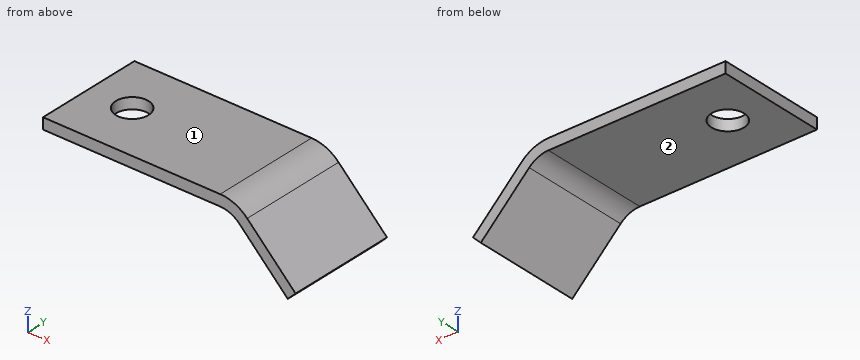
Autodesk Inventor part; units mm, degrees
ref_plane "YZ Plane" through (0, 0, 0) normal (1, 0, 0) x (0, 1, 0)
ref_plane "XZ Plane" through (0, 0, 0) normal (0, 1, 0) x (-1, 0, 0)
ref_plane "XY Plane" through (0, 0, 0) normal (0, 0, 1) x (1, 0, 0)
sketch "Sketch1" plane through (0, 0, 0) normal (0, 1, 0) x (-1, 0, 0)
  line L0 (0, 0) -> (-5.4801, -5.4801)
  line L1 (0, 0) -> (17.75, 0)
  dimension "d0" = 7.75
  dimension "d2" = 17.75
  dimension "d3" = 135
contour flange "Contour Flange1" sketch "Sketch1" thickness 1.016 bend radius 2.5 width 10 along (0, 1, 0) mid plane no both sides no wall seen from (2.74, 0, -2.74) lies toward (-0.7071068, 0, -0.7071068) curves L0 L1
bend "Bend1"
corner "Corner1"
sketch "Sketch2" plane through (-17.75, 0, -1.016) normal (0, 0, -1) x (-1, 0, 0)
  point P0 (-17.75, 0)
  point P1 (0, 0)
  point P2 (-4, 5)
  dimension "d15" = 5
  dimension "d16" = 4
hole "Hole1" at (-13.75, 5, -1.016) direction (0, 0, 1) diameter 3 end through all
equation "\"d22\" = Thickness"
equation "\"d4\" = Thickness"
equation "\"d5\" = BendReliefWidth"
equation "\"d6\" = BendReliefDepth"
equation "\"d7\" = MinimumRemnant"
equation "\"d8\" = TransitionRadius"
equation "\"d12\" = CornerReliefSize"
equation "\"d13\" = GapSize"
equation "\"d14\" = JacobiRadiusSize"
equation "\"BendRadius\" = Thickness"
equation "\"BendReliefWidth\" = Thickness"
equation "\"BendReliefDepth\" = 0.5 * Thickness"
equation "\"CornerReliefSize\" = 4 * Thickness"
equation "\"MinimumRemnant\" = 2 * Thickness"
equation "\"TransitionRadius\" = BendRadius"
equation "\"JacobiRadiusSize\" = BendRadius"
equation "\"GapSize\" = Thickness"
properties part number "Piston Flag" material "ABS Plastic"
Can you work these out from the model? Positions are in its coordinate system, mm. Face numbers are marked on the shaded views. A direction names the side the tool comes from. Coordinates: 2 decimals unless noted, no trailing zeros. Loops run counter-clockwise (first coordinate to the right, second up) from the corner with the lowest first, then second, coordinate; pieces in that order, holes last. Notation, with made-up numbers: (8.5, 72) - (51.5, 72) arc R14 ccw to (51.5, 82) - close; hole circle Ø6 at (-18.75, 24.25). An arc over 180 degrees is marked (long way). Answer as CSV lines item,"result". Start each with the question number.
1) Which directions (+Z, -Z, +X, -X, +Y, -Y) give clear straight access to the entire face, cutting with the end or side of a thin tool? Please do the marked faces 1 and 2.
2) Suppose I cut it at D-D (z = -3.25). Please give me the cut outline in (x, y).
3) Suppose I cut it at A-A (y = 5). Please give me the cut outline in (x, z), plus the area to 3 significant figures.
4) Suppose I cut it at B-B (x = -13.75). Please give me the cut outline in (y, z), plus the area to 3 significant figures.
5) For pin 1 (1.8 mm diameter, centred on x = -13.75, y = 5, fed in from +Z); pin 2 (1 mm diameter, centred on x = -11.5, y = 7.5, fed in from +Z); pin 3 (6 mm diameter, centred on x = -5, y = 2.5, fed in from -Z); pin 4 (2 mm diameter, centred on x = 1, y = 6, fed in from +Z), each with a flat end and sliding along its axis, tell me the tip position at first contact or that it passes through.
6) I need wall thicknesses on line 1 (Y direction, x = -13.75, z = -0.35); line 2 (Z direction, x = -11.75, y = 3); line 3 (X direction, y = 5, z = -0.8). Which ranges of each line are inside material? Lowest first, please. Write a range as from..to.
7) Suppose I cut it at C-C (y = 0.5). Please give me the cut outline in (x, z), plus the area to 3 significant figures.
Check result:
1,face 1,"+Z, +X, -X, +Y, -Y"
1,face 2,"-Z, -X, +Y, -Y"
2,outline,"(1.81, 0) - (3.25, 0) - (3.25, 10) - (1.81, 10) - close"
3,outline,"(-17.75, -1.02) - (-15.25, -1.02) - (-15.25, 0) - (-17.75, 0) - close; (-12.25, -1.02) - (-1.46, -1.02) arc R2.5 cw to (0.31, -1.75) - (4.76, -6.2) - (5.48, -5.48) - (1.03, -1.03) arc R3.52 ccw to (-1.46, 0) - (-12.25, 0) - close"
3,area,"22.3 mm²"
4,outline,"(0, -1.02) - (3.5, -1.02) - (3.5, 0) - (0, 0) - close; (6.5, -1.02) - (10, -1.02) - (10, 0) - (6.5, 0) - close"
4,area,"7.11 mm²"
5,pin 1,"passes through"
5,pin 2,"stops at z = 0"
5,pin 3,"stops at z = -1.02"
5,pin 4,"stops at z = -0.32"
6,line 1,"y = 0..3.5, 6.5..10"
6,line 2,"z = -1.02..0"
6,line 3,"x = -17.75..-15.25, -12.25..0.78"
7,outline,"(-17.75, -1.02) - (-1.46, -1.02) arc R2.5 cw to (0.31, -1.75) - (4.76, -6.2) - (5.48, -5.48) - (1.03, -1.03) arc R3.52 ccw to (-1.46, 0) - (-17.75, 0) - close"
7,area,"25.3 mm²"
